The model under review builds one solid part; all positions refer to its coordinate system, in mm. A direction names the side the tool comes from. Coordinates: 2 decimals unless noted, no trailing zeros. Order: outer loops, then holes, each group sorted by start corner. A loop starts at its lowest first (then second) coordinate and runs counter-clockwise, first axis right, second up. Notation, with made-up numbers: M -31,25.25 L 16,25.25 A27 cw 16,50.25 Z; hole C 77.25,56.25 d7. An arc over 180 degrees is marked long. Answer in a Markdown table with one row per item.
Autodesk Inventor part; units mm, degrees
ref_plane "YZ Plane" through (0, 0, 0) normal (1, 0, 0) x (0, 1, 0)
ref_plane "XZ Plane" through (0, 0, 0) normal (0, 1, 0) x (-1, 0, 0)
ref_plane "XY Plane" through (0, 0, 0) normal (0, 0, 1) x (1, 0, 0)
sketch "Sketch1" plane through (0, 0, 0) normal (0, 1, 0) x (-1, 0, 0)
  circle A0 centre (8, 0) radius 1.5
  circle A1 centre (-8, 0) radius 1.5
  line L0 (12, -3) -> (-12, -3)
  line L1 (-12, -3) -> (-12, 3)
  line L2 (-12, 3) -> (12, 3)
  line L3 (12, 3) -> (12, -3)
  circle A2 centre (0, 0) radius 1.4
  circle A3 centre (0, 0) radius 3
  point P0 (-12, 0)
  point P1 (0, 3)
  dimension "d0" = 3
  dimension "d1" = 3
  dimension "d2" = 8
  dimension "d3" = 8
  dimension "d4" = 24
  dimension "d5" = 6
  dimension "d6" = 2.8
extrude "Extrusion1" add sketch "Sketch1" along normal blind 2 contours L0 A3 L2 L3 | L0 L1 L2 A3 | A3 | A2
extrude "Extrusion2" add sketch "Sketch1" against normal blind 8 contours A3
fillet "Fillet2" radius 2 4 edges at (-12, 1, 3) (-12, 1, -3) (12, 1, 3) (12, 1, -3)
properties part number "Shaft Encoder Adapter" material "ABS Plastic"
(1) Machinability: for faces 5 (the cylindrical face through (1.4, -3.94, 0.06)), 6 (the cylindrical face through (11.4, 1.01, 2.43)), which of the approach directions +Z, -Z, +X, -X, +Y, -Y give a long, thin tool a straight path to every point of the face, cutting with its end or side? Answer none if there is none.
Report:
| item | result |
|---|---|
| face 5 | -Y |
| face 6 | +Z, +X, +Y, -Y |
(2) Take a section at C-C (y = -1). Write out the cut boundary in (x, z).
Report:
| item | result |
|---|---|
| outline | C 0,0 d6; hole C 0,0 d2.8 |
(3) Insertion check: P1, Ø1, axis at y = -3, z = 0, coming from the +X side; P2, Ø1.7, axis at x = 0, z = 0, coming from the -Y side; P3, Ø2, axis at x = 4.5, y = -4.5, coming from the -Z side. Each pin has a flat end and moves straight along its axis. Give the tip position at first contact, or say it passes through.
Report:
| item | result |
|---|---|
| P1 | x = 3 |
| P2 | y = 0 |
| P3 | through |
(4) Take a section at A-A (z = 0). Write out the cut boundary in (x, y).
Report:
| item | result |
|---|---|
| outline | M -12,0 L -9.5,0 L -9.5,2 L -12,2 Z; M -6.5,0 L -3,0 L -3,-8 L -1.4,-8 L -1.4,0 L 1.4,0 L 1.4,-8 L 3,-8 L 3,0 L 6.5,0 L 6.5,2 L -6.5,2 Z; M 9.5,0 L 12,0 L 12,2 L 9.5,2 Z |
(5) To check wall thickness, follow line 1 (X direction, y = 0.25, z = 1); line 2 (Z direction, x = 8, y = 1.3); line 3 (Y direction, x = 7.5, z = 2.75). State the ranges of each line that lie inside material, in increasing order. Write a range as [from, to].
Report:
| item | result |
|---|---|
| line 1 | [-12, -9.12], [-6.88, 6.88], [9.12, 12] |
| line 2 | [-3, -1.5], [1.5, 3] |
| line 3 | [0, 2] |
(6) Take a section at B-B (x = 8). Write out the cut boundary in (y, z), then the cut area to 3 significant figures.
Report:
| item | result |
|---|---|
| outline | M 0,-3 L 2,-3 L 2,-1.5 L 0,-1.5 Z; M 0,1.5 L 2,1.5 L 2,3 L 0,3 Z |
| area | 6.00 mm^2 |
(7) Take a section at D-D (x = -9). Write out the cut boundary in (y, z), then the cut area to 3 significant figures.
Report:
| item | result |
|---|---|
| outline | M 0,-3 L 2,-3 L 2,-1.12 L 0,-1.12 Z; M 0,1.12 L 2,1.12 L 2,3 L 0,3 Z |
| area | 7.53 mm^2 |
(8) The part is to be moulded in two halves that separate along Z. For faces 1 (the cylindrical face through (-6.5, 0.99, -0.07)), 2 (the cylindrical face through (9.5, 0.99, -0.07)), 3 (the flat face through (0, 1, -3)), 4 (the flat face through (-12, 1, 0)), say which applies: +Z half, -Z half, draft (parallel to the pull), parting line (faces both ways), or undercut.
Report:
| item | result |
|---|---|
| face 1 | undercut |
| face 2 | undercut |
| face 3 | -Z half |
| face 4 | draft |
